from build123d import *

# Parameters (mm, degrees)
SKETCH1_R           = 5
BOSS_EXTRUDE1_DEPTH = 2.2


with BuildPart() as part:
    # Sketch1 → Boss-Extrude1 (new body)
    with BuildSketch(Plane(origin=(0, 0, 0), x_dir=(1, 0, 0), z_dir=(0, 1, 0))):
        Polygon((-154.536383046, 11.329521193), (-146.536383046, 11.329521193), (-146.536383046, 13.329521193), (-138.536383046, 13.329521193), (-138.536383046, 16.329521193), (-138.536383046, 22.329521193), (-140.036383046, 22.329521193), (-140.036383046, 30.329521193), (-138.536383046, 30.329521193), (-138.536383046, 36.329521193), (-138.536383046, 37.509521193), (-147.536383046, 37.509521193), (-147.536383046, 36.329521193), (-153.536383046, 36.329521193), (-153.536383046, 37.509521193), (-162.536383046, 37.509521193), (-162.536383046, 36.329521193), (-162.536383046, 13.329521193), (-154.536383046, 13.329521193), align=None)
        with Locations(Location((-150.536383046, 23.829521193, 0), (0, 0, 270))):
            Circle(SKETCH1_R, mode=Mode.SUBTRACT)
    extrude(amount=BOSS_EXTRUDE1_DEPTH)


solid = part.part
Read the model definition and answer for the solid it produces. Units are mm, in the model's axes. A direction names the side the tool comes from. Round coordinates to 2 decimals unless told otherwise and drop trailing zeros. Write each loop counter-clockwise with the first axis right and the second up, starting at its lowest first coordinate (ties: lowest second). Pieces come first, ordered by that corner, then holes. Notation, with made-up numbers: (-5, 26.5) - (43, 26.5) arc R21 cw to (43, 45.5) - close; hole circle Ø9 at (66, -4.75). An arc over 180 degrees is marked (long way). One line per question, with ' | ' between items. Start each with the question number.
1. Section A-A (y = 1.6) is taken. Determine the outline of the cut face in (x, z), and give its area (3 significant figures).
2. Find the intervals of material crossed by probe 1 along X at (y, z) = (1, -36.5); probe 2 along Z at (x, y) = (-154.5, 1); probe 3 along Z at (x, y) = (-159.25, 1.6), in increasing order. Write a range as [from, to].
3. For a pull along X with two mould halves and no side action, classify faces 1 (the face through (-153.536, 1, -37)), 2 (the face through (-140.036, 1, -26)), 3 (the face through (-154.536, 1, -12)), 4 (the face through (-147.536, 1, -37)) as +X half, -X half, draft (parallel to the pull), parting line (faces both ways), or undercut.
4. For faces 5 (the face through (-146.536, 1, -12)), 6 (the face through (-150, 1, -36.33)), 7 (the face through (-158, 1, -37.51)), 8 (the face through (-159, 1, -13.33)), 9 (the face through (-139, 1, -22.33)), determine the directions among +Z, -Z, +X, -X, +Y, -Y from which every point of the face is accessible in a straight line to the end or side of a thin tool.
5. Section B-B (z = -24.25) is taken. Determine the outline of the cut face in (x, y), and give its area (3 significant figures).
6. Each of these flat-tipped pins is pushed along its axis until it touches: pin 1 (0.6 mm diameter, centred on y = 0.5, z = -12.5, fed in from +X); pin 2 (1.1 mm diameter, centred on x = -150.5, y = 1.5, fed in from -Z); pin 3 (0.8 mm diameter, centred on x = -139.5, y = 0.5, fed in from +Z); pin 4 (9 mm diameter, centred on x = -150.54, z = -23.83, fed in from +Y). Where does it stop, or does it pass through?
7. Section C-C (x = -159.25) is taken. Determine the outline of the cut face in (y, z), and give its area (3 significant figures).
Filled in:
1) outline: (-162.54, -37.51) - (-153.54, -37.51) - (-153.54, -36.33) - (-147.54, -36.33) - (-147.54, -37.51) - (-138.54, -37.51) - (-138.54, -30.33) - (-140.04, -30.33) - (-140.04, -22.33) - (-138.54, -22.33) - (-138.54, -13.33) - (-146.54, -13.33) - (-146.54, -11.33) - (-154.54, -11.33) - (-154.54, -13.33) - (-162.54, -13.33) - close; hole circle Ø10 at (-150.54, -23.83) | area: 499 mm²
2) probe 1: [-162.54, -153.54], [-147.54, -138.54] | probe 2: [-37.51, -26.88], [-20.78, -11.33] | probe 3: [-37.51, -13.33]
3) face 1: undercut | face 2: +X half | face 3: -X half | face 4: undercut
4) face 5: +Z, +X, +Y, -Y | face 6: -Z, +Y, -Y | face 7: -Z, +X, -X, +Y, -Y | face 8: +Z, -X, +Y, -Y | face 9: +X, +Y, -Y
5) outline: (-162.54, 0) - (-155.52, 0) - (-155.52, 2.2) - (-162.54, 2.2) - close; (-145.55, 0) - (-140.04, 0) - (-140.04, 2.2) - (-145.55, 2.2) - close | area: 27.6 mm²
6) pin 1: x = -146.54 | pin 2: z = -36.33 | pin 3: z = -13.33 | pin 4: through
7) outline: (0, -37.51) - (2.2, -37.51) - (2.2, -13.33) - (0, -13.33) - close | area: 53.2 mm²
